```python
from build123d import *

# Parameters (mm, degrees)
SKETCH_W        = 60
SKETCH_H        = 60
SKETCH_W_2      = 54
SKETCH_H_2      = 54
PAD_DEPTH       = 120
SKETCH001_R     = 2.75
POCKET_DEPTH    = 3
SKETCH002_R     = 2.75
POCKET001_DEPTH = 3
SKETCH003_R     = 3
POCKET002_DEPTH = 3


with BuildPart() as part:
    # Sketch → Pad (new body)
    with BuildSketch(Plane.XZ):
        Rectangle(SKETCH_W, SKETCH_H)
        Rectangle(SKETCH_W_2, SKETCH_H_2, mode=Mode.SUBTRACT)
    extrude(amount=PAD_DEPTH)

    # Sketch001 (on Face3 of Pad) → Pocket (cut)
    with BuildSketch(Plane(origin=(0, 0, -30), x_dir=(1, 0, 0), z_dir=(0, 0, -1))):
        with Locations((-19, 108)):
            Circle(SKETCH001_R)
        with Locations((-19, 78)):
            Circle(SKETCH001_R)
        with Locations((19, 108)):
            Circle(SKETCH001_R)
        with Locations((19, 78)):
            Circle(SKETCH001_R)
        with Locations((-19, 42)):
            Circle(SKETCH001_R)
        with Locations((-19, 12)):
            Circle(SKETCH001_R)
        with Locations((19, 42)):
            Circle(SKETCH001_R)
        with Locations((19, 12)):
            Circle(SKETCH001_R)
    extrude(amount=-POCKET_DEPTH, mode=Mode.SUBTRACT)

    # Sketch002 (on Face1 of Pocket) → Pocket001 (cut)
    with BuildSketch(Plane(origin=(0, 0, 30), x_dir=(-1, 0, 0), z_dir=(0, 0, 1))):
        with Locations((-20, 46)):
            Circle(SKETCH002_R)
        with Locations((-20, 22)):
            Circle(SKETCH002_R)
        with Locations((20, 46)):
            Circle(SKETCH002_R)
        with Locations((20, 22)):
            Circle(SKETCH002_R)
    extrude(amount=-POCKET001_DEPTH, mode=Mode.SUBTRACT)

    # Sketch003 (on Face5 of Pocket001) → Pocket002 (cut)
    with BuildSketch(Plane(origin=(30, 0, 0), x_dir=(0, 0, 1), z_dir=(1, 0, 0))):
        with Locations((-20, 110)):
            Circle(SKETCH003_R)
        with Locations((20, 110)):
            Circle(SKETCH003_R)
        with Locations((-20, 70)):
            Circle(SKETCH003_R)
        with Locations((20, 70)):
            Circle(SKETCH003_R)
    extrude(amount=-POCKET002_DEPTH, mode=Mode.SUBTRACT)


solid = part.part
```
Can you work these out from the model? Positions are in its coordinate system, mm. A direction names the side the tool comes from. Coordinates: 2 decimals unless noted, no trailing zeros. Order: outer loops, then holes, each group sorted by start corner. A loop starts at its lowest first (then second) coordinate and runs counter-clockwise, first axis right, second up.
1. Thinking about a two-plate mould opening in X: for faces 5 (the face through (-2, 0, -29)), 6 (the face through (0, -59, -27)), 7 (the face through (22.747, -22.121, 28.521)), 8 (the face through (-30, -59, 0)), which applies, +X half, -X half, draft (parallel to the pull), parting line (faces both ways), or undercut?
2. I'm going to push flat-ended pins straight in: pin 1 (5 mm diameter, centred on x = -19, y = -12, fed in from -Z); pin 2 (3.5 mm diameter, centred on y = -70, z = -20, fed in from +X). Where does each tip first touch, or does it pass through?
3. For faces 1 (the face through (28.5, -108.2, -22.4)), 2 (the face through (-27, -59, 0)), 3 (the face through (20.358, -48.727, 28.521)), 4 (the face through (-19.358, -44.727, -28.521)), which set-ups out of +Z, -Z, +X, -X, +Y, -Y let a thin tool reach every point of the face, with its end or its side?
4. If we section it at B-B (y = -96): Please give me the cut outline in (x, z), then the cut area to 3 significant figures.
5. I need wall thicknesses on line 1 (Y direction, x = 19, z = -29.05); line 2 (X direction, y = -78, z = -28.45); line 3 (Z direction, x = 28.6, y = -110). Which ranges of each line are inside material? Lowest first, please.
6. If we section it at D-D (y = -22): Please give me the cut outline in (x, z), then the cut area to 3 significant figures.
7. If we section it at A-A (z = -8): Please give me the cut outline in (x, y), then the cut area to 3 significant figures.
8. If we section it at C-C (x = -2.5): Please give me the cut outline in (y, z).
Entries:
1. face 5: draft
1. face 6: undercut
1. face 7: undercut
1. face 8: -X half
2. pin 1: stops at z = 27
2. pin 2: stops at x = -27
3. face 1: +X
3. face 2: +Y, -Y
3. face 3: +Z
3. face 4: -Z
4. outline: (-30, -30) - (30, -30) - (30, 30) - (-30, 30) - close; hole (-27, -27) - (27, -27) - (27, 27) - (-27, 27) - close
4. area: 684 mm2
5. line 1: y = -120 to -110.75, -105.25 to -80.75, -75.25 to -44.75, -39.25 to -14.75, -9.25 to 0
5. line 2: x = -30 to -21.75, -16.25 to 16.25, 21.75 to 30
5. line 3: z = -30 to -23, -17 to 17, 23 to 30
6. outline: (-30, -30) - (30, -30) - (30, 30) - (22.75, 30) - (22.75, 27) - (27, 27) - (27, -27) - (-27, -27) - (-27, 27) - (-22.75, 27) - (-22.75, 30) - (-30, 30) - close; (-17.25, 27) - (17.25, 27) - (17.25, 30) - (-17.25, 30) - close
6. area: 651 mm2
7. outline: (-30, -120) - (-27, -120) - (-27, 0) - (-30, 0) - close; (27, -120) - (30, -120) - (30, 0) - (27, 0) - close
7. area: 720 mm2
8. outline: (-120, -30) - (0, -30) - (0, -27) - (-120, -27) - close; (-120, 27) - (0, 27) - (0, 30) - (-120, 30) - close
